CAD build for the part. Positions are in the model's coordinates, mm. A direction names the side the tool comes from. Give positions to 0.01 mm unless a question says otherwise; leave off trailing zeros. Order: outer loops, then holes, each group sorted by start corner. A loop starts at its lowest first (then second) coordinate and runs counter-clockwise, first axis right, second up.
```python
from build123d import *

# Parameters (mm, degrees)
F0_W     = 50.8
F0_H     = 42.9
F0_R     = 1
F0_R_2   = 1.6
F0_R_3   = 5
F0_R_4   = 2.2
F1_DEPTH = 3
F2_R     = 1
F3_W     = 3
F3_H     = 5
F3_H_2   = 4
F3_W_2   = 5
F3_H_3   = 3
F4_DEPTH = 4
F5_SIZE  = 1.5
F6_SIZE  = 2.99999
F7_SIZE  = 2.99999


# Not quite as in the source:
# - a fillet or chamfer is up to 0.001 mm smaller than in the source, because OpenCascade refuses the exact size


with BuildPart() as f1:
    # F0 (on Front) → F1 (new body)
    with BuildSketch(Plane.XZ):
        Rectangle(F0_W, F0_H)
        with Locations((0, -17.25)):
            Circle(F0_R, mode=Mode.SUBTRACT)
        with Locations((-7.7781745931, -7.7781745931)):
            Circle(F0_R, mode=Mode.SUBTRACT)
        with Locations((0, -9.5)):
            Circle(F0_R_2, mode=Mode.SUBTRACT)
        with BuildLine():
            ThreePointArc((21.4, -15.45), (20.8142135624, -16.8642135624), (19.4, -17.45))
            Line((19.4, -17.45), (15.4, -17.45))
            ThreePointArc((15.4, -17.45), (13.9857864376, -16.8642135624), (13.4, -15.45))
            Line((13.4, -15.45), (13.4, -11.45))
            ThreePointArc((13.4, -11.45), (13.9857864376, -10.0357864376), (15.4, -9.45))
            Line((15.4, -9.45), (19.4, -9.45))
            ThreePointArc((19.4, -9.45), (20.8142135624, -10.0357864376), (21.4, -11.45))
            Line((21.4, -11.45), (21.4, -15.45))
        make_face(mode=Mode.SUBTRACT)
        with Locations((7.7781745931, -7.7781745931)):
            Circle(F0_R, mode=Mode.SUBTRACT)
        with Locations((-17.25, 0)):
            Circle(F0_R, mode=Mode.SUBTRACT)
        with Locations((-9.5, 0)):
            Circle(F0_R_2, mode=Mode.SUBTRACT)
        Circle(F0_R_3, mode=Mode.SUBTRACT)
        with Locations((-7.7781745931, 7.7781745931)):
            Circle(F0_R, mode=Mode.SUBTRACT)
        with Locations((0, 9.5)):
            Circle(F0_R_2, mode=Mode.SUBTRACT)
        with Locations((-12.7, 17.5)):
            Circle(F0_R_4, mode=Mode.SUBTRACT)
        with Locations((0, 17.25)):
            Circle(F0_R, mode=Mode.SUBTRACT)
        with Locations((9.5, 0)):
            Circle(F0_R_2, mode=Mode.SUBTRACT)
        with Locations((7.7781745931, 7.7781745931)):
            Circle(F0_R, mode=Mode.SUBTRACT)
        with Locations((17.25, 0)):
            Circle(F0_R, mode=Mode.SUBTRACT)
        with Locations((12.7, 17.5)):
            Circle(F0_R_4, mode=Mode.SUBTRACT)
    extrude(amount=F1_DEPTH)

    # F2
    f2_edges = [f1.edges().sort_by_distance(p)[0] for p in [
        (25.4, -1.5, 21.45),
        (25.4, -1.5, -21.45),
        (-25.4, -1.5, -21.45),
        (-25.4, -1.5, 21.45),
    ]]
    fillet(f2_edges, radius=F2_R)

    # F3 (on face) → F4 (join)
    with BuildSketch(Plane(origin=(0, 0, 0), x_dir=(-1, 0, 0), z_dir=(0, 1, 0))):
        with Locations((-18.9, 13.95)):
            Rectangle(F3_W, F3_H)
        with Locations((-18.9, -7.45)):
            Rectangle(F3_W, F3_H_2)
        with Locations((18.9, 13.95)):
            Rectangle(F3_W, F3_H)
        Polygon((20.4, -16.45), (20.4, -5.45), (17.4, -5.45), (17.4, -13.45), (8.4, -13.45), (8.4, -16.45), align=None)
        with Locations((-10.9, -14.95)):
            Rectangle(F3_W_2, F3_H_3)
    extrude(amount=F4_DEPTH)

    # F5
    f5_edges = [f1.edges().sort_by_distance(p)[0] for p in [
        (13.4, 2, -13.45),
        (17.4, 2, -9.45),
    ]]
    chamfer(f5_edges, length=F5_SIZE)

    # F6 (size 3 in the source; OpenCascade refuses exactly that, so slightly less here)
    f6_edges = [f1.edges().sort_by_distance(p)[0] for p in [
        (17.4, 4, 13.95),
    ]]
    chamfer(f6_edges, length=F6_SIZE)

    # F7 (size 3 in the source; OpenCascade refuses exactly that, so slightly less here)
    f7_edges = [f1.edges().sort_by_distance(p)[0] for p in [
        (-17.4, 4, 13.95),
        (-17.4, 4, -9.45),
        (-12.9, 4, -13.45),
        (10.15, 4, -13.45),
        (17.4, 4, -6.7),
    ]]
    chamfer(f7_edges, length=F7_SIZE)


solid = f1.part
```
Item 1: Slice it at C-C (y = 3.25). Give the cut face in (x, z).
Item 2: Two-plate mould, pull along Z, no slides. Class faces 1 (the face through (20.83, -1.48, -16.85)), 2 (the face through (18.31, 0.95, -8.86)), 3 (the face through (19, 2, 16.45)): released by +Z, released by -Z, zero draft, split by the parting line, or undercut.
Item 3: Slice it at D-D (y = -1.25). State how many separate pieces and enclosed holes the cut face has, and give its area (3 significant figures).
Item 4: Slice it at B-B (z = 3). Give the cut face in (x, y).
Item 5: Tool access for faces 4 (the face through (-8.4, 2, -15)), 5 (the face through (19, 2, 11.45)), 6 (the face through (14, -1.48, -16.88)): list every direction of +Z, -Z, +X, -X, +Y, -Y with a clear straight run to the whole face (end or side of a thin tool).
Item 6: Wall check: L1, parallel to X at y = 0.25, z = 12; L2, parallel to Z at x = 0, y = -2.25; L3, parallel to X at y = -2, z = -10. Give the ranges that are in metal, low to high.
Item 7: Drop flat-ended pins along their axis: pin 1 Ø3 at (x, y) = (-12.5, 3) entering from -Z; pin 2 Ø21.5 at (x, z) = (-8, 0.5) entering from +Y; pin 3 Ø3.5 at (x, y) = (18.5, 2) entering from +Z. Give the stop position or say it passes through.
A:
1. outline: (-20.4, -16.45) - (-8.4, -16.45) - (-8.4, -15.7) - (-19.65, -15.7) - (-19.65, -5.45) - (-20.4, -5.45) - close; (-20.4, 11.45) - (-19.65, 11.45) - (-19.65, 16.45) - (-20.4, 16.45) - close; (8.4, -16.45) - (13.4, -16.45) - (13.4, -15.7) - (8.4, -15.7) - close; (19.65, -9.45) - (20.4, -9.45) - (20.4, -5.45) - (19.65, -5.45) - close; (19.65, 11.45) - (20.4, 11.45) - (20.4, 16.45) - (19.65, 16.45) - close
2. face 1: undercut
2. face 2: released by -Z
2. face 3: released by +Z
3. separate pieces: 1
3. enclosed holes: 16
3. area: 1,950 mm2
4. outline: (-25.4, -3) - (-4, -3) - (-4, 0) - (-25.4, 0) - close; (4, -3) - (25.4, -3) - (25.4, 0) - (4, 0) - close
5. face 4: +Z, -Z, +Y
5. face 5: +X, -X, +Y
5. face 6: +Y, -Y
6. L1: x = -20.4 to -17.4, 17.4 to 20.4
6. L2: z = -21.45 to -18.25, -16.25 to -11.1, -7.9 to -5, 5 to 7.9, 11.1 to 16.25, 18.25 to 21.45
6. L3: x = -25.4 to -1.52, 1.52 to 14.02, 20.78 to 25.4
7. pin 1: stops at z = -16.45
7. pin 2: stops at y = 0
7. pin 3: stops at z = 16.45
